```python
from build123d import *

# Parameters (mm, degrees)
PAD_DEPTH       = 23
POCKET_DEPTH    = 20
SKETCH002_R     = 3
PAD001_DEPTH    = 5
SKETCH003_R     = 1.75
POCKET001_DEPTH = 7
SKETCH004_R     = 7
POCKET002_DEPTH = 37


with BuildPart() as part:
    # Sketch (on Face1 of ShapeBinder) → Pad (new body)
    with BuildSketch(Plane.XY.offset(1.6)):
        with BuildLine():
            Line((65.104061, -85.85), (78.671175, -85.849875))
            ThreePointArc((78.671175, -85.849875), (81.499513, -84.678339), (82.67105, -81.850001))
            ThreePointArc((85.065002, -79.425001), (83.370362, -80.146209), (82.67105, -81.850001))
            Line((85.065002, -79.425001), (184.315, -79.425))
            Line((184.315, -79.425), (184.315, -33.325))
            Line((184.315, -33.325), (85.065, -33.325))
            Line((85.065, -33.325), (66.055583, -33.325))
            Line((66.055583, -33.325), (58.318648, -33.167991))
            ThreePointArc((58.318648, -33.167991), (41.347688, -32.282578), (32.59625, -46.85))
            Line((32.59625, -46.85), (32.59625, -81.85))
            ThreePointArc((32.59625, -81.85), (47.081166, -98.22649), (65.104061, -85.85))
        make_face()
    extrude(amount=PAD_DEPTH)

    # Sketch001 (on Face11 of Pad) → Pocket (cut)
    with BuildSketch(Plane.XY.offset(24.6)):
        with BuildLine():
            Line((85.065004, -76.42489), (181.315, -76.425))
            Line((181.315, -76.425), (181.315, -36.325))
            Line((181.315, -36.325), (66.055583, -36.325))
            ThreePointArc((66.055583, -36.325), (66.025147, -36.324846), (65.994715, -36.324382))
            Line((65.994715, -36.324382), (58.25778, -36.167373))
            ThreePointArc((58.25778, -36.167373), (57.41292, -36.028001), (56.641848, -35.655629))
            ThreePointArc((56.641848, -35.655629), (42.756517, -34.9312), (35.59625, -46.85))
            Line((35.59625, -46.85), (35.59625, -81.85))
            ThreePointArc((35.59625, -81.85), (47.447597, -95.248953), (62.193575, -85.122625))
            ThreePointArc((62.193575, -85.122625), (63.25771, -83.485372), (65.104092, -82.849876))
            Line((65.104092, -82.849876), (78.671175, -82.849878))
            ThreePointArc((78.671175, -82.849878), (79.378193, -82.557021), (79.67105, -81.850003))
            ThreePointArc((85.065004, -76.42489), (81.249022, -78.024869), (79.67105, -81.850003))
        make_face()
    extrude(amount=-POCKET_DEPTH, mode=Mode.SUBTRACT)

    # Sketch002 (on Face26 of Pocket) → Pad001 (join)
    with BuildSketch(Plane.XY.offset(4.6)):
        with Locations((64.665, -78.375)):
            Circle(SKETCH002_R)
        with Locations((49.065, -64.325)):
            Circle(SKETCH002_R)
        with Locations((60.665, -41.375)):
            Circle(SKETCH002_R)
        with Locations((104.065, -56.325)):
            Circle(SKETCH002_R)
        with Locations((123.165, -56.375)):
            Circle(SKETCH002_R)
        with Locations((142.215, -56.375)):
            Circle(SKETCH002_R)
        with Locations((161.265, -56.375)):
            Circle(SKETCH002_R)
    extrude(amount=PAD001_DEPTH)

    # Sketch003 (on Face37 of Pad001) → Pocket001 (cut)
    with BuildSketch(Plane.XY.offset(9.6)):
        with Locations((49.065, -64.325)):
            Circle(SKETCH003_R)
        with Locations((64.665, -78.375)):
            Circle(SKETCH003_R)
        with Locations((60.665, -41.375)):
            Circle(SKETCH003_R)
        with Locations((142.215, -56.375)):
            Circle(SKETCH003_R)
        with Locations((161.265, -56.375)):
            Circle(SKETCH003_R)
        with Locations((104.065, -56.325)):
            Circle(SKETCH003_R)
        with Locations((123.165, -56.375)):
            Circle(SKETCH003_R)
    extrude(amount=-POCKET001_DEPTH, mode=Mode.SUBTRACT)

    # Sketch004 → Pocket002 (cut)
    with BuildSketch(Plane.XZ):
        with Locations((72.507256, 16.6)):
            Circle(SKETCH004_R)
    extrude(amount=POCKET002_DEPTH, mode=Mode.SUBTRACT)


solid = part.part
```
Source: CAD feature listing. Evaluate the final solid. Frame: model axes, mm. A direction names the side the tool comes from. Coordinates: 2 decimals unless noted, no trailing zeros. Loops run counter-clockwise (first coordinate to the right, second up) from the corner with the lowest first, then second, coordinate; pieces in that order, holes last. Notation, with made-up numbers: M -3.75,-33 L 38.25,-33 A26 cw 38.25,3 Z; hole C 77,13 d6. An arc over 180 degrees is marked long. Put each result on its own line as item: value. Start each with the question number.
1) Cut plane B-B on z = 16.6. Return the cut outline in (x, y) (3 decimals), then the cut area to 3 significant figures.
2) Reachability of faces 1 (the face through (65.514, -34.797, 16.908)), 2 (the face through (46.75, -98.182, 12.939)), 3 (the face through (144, -58, 9.6)), 4 (the face through (126, -33.325, 13)) from +Z, -Z, +X, -X, +Y, -Y: full face, straight path, thin tool, end or side. Return the list, or none.
3) Cut plane A-A on y = -51.5. Return the cut outline in (x, z) (3 decimals), then the cut area to 3 significant figures.
4) Cut plane C-C on x = 128. Return the cut outline in (y, z) (3 decimals), then the cut area to 3 significant figures.
5) Pull-direction query (Y, two-part tool) for faces 5 (the face through (97, -77, 24.6)), 6 (the face through (81.47, -84.71, 12.94)), 7 (the face through (41.569, -32.167, 12.939)), 8 (the face through (65, -78, 2.6)); classes: pulls with the +Y half, pulls with the -Y half, needs draft (parallel to the pull), parting line crosses it, or undercut.
6) Contact query for flat-ended pins moving along their axis: pin 1 Ø10 at (x, z) = (113.5, 10) entering from -Y (3 decimals); pin 2 Ø5 at (x, y) = (160, -56) entering from +Z; pin 3 Ø1 at (x, y) = (143, -56.5) entering from +Z. Output: stop coordinate, or through.
7) Ray query, L1, parallel to Y at x = 134.5, z = 22.5 (3 decimals); L2, parallel to X at y = -69, z = 21.5 (3 decimals); L3, parallel to X at y = -35, z = 14 (3 decimals). Return the intervals inside material, ascending. Write a range as from..to.
The answers:
1. outline: M 32.596,-81.85 A16.5 ccw 65.104,-85.85 L 78.671,-85.85 A4 ccw 82.671,-81.85 A2.425 cw 85.065,-79.425 L 184.315,-79.425 L 184.315,-33.325 L 79.507,-33.325 L 79.507,-36.325 L 181.315,-36.325 L 181.315,-76.425 L 85.065,-76.425 A5.425 ccw 79.671,-81.85 A1 cw 78.671,-82.85 L 65.104,-82.85 A3 ccw 62.194,-85.123 A13.5 cw 35.596,-81.85 L 35.596,-46.85 A13.5 cw 56.642,-35.656 A3 ccw 58.258,-36.167 L 65.507,-36.314 L 65.507,-33.314 L 58.319,-33.168 A16.5 ccw 32.596,-46.85 Z
1. area: 1,170 mm²
2. face 1: +Y
2. face 2: +Z, -Z, -Y
2. face 3: +Z
2. face 4: +Z, -Z, +X, +Y
3. outline: M 32.596,1.6 L 184.315,1.6 L 184.315,24.6 L 181.315,24.6 L 181.315,4.6 L 35.596,4.6 L 35.596,24.6 L 32.596,24.6 Z
3. area: 575 mm²
4. outline: M -79.425,1.6 L -33.325,1.6 L -33.325,24.6 L -36.325,24.6 L -36.325,4.6 L -76.425,4.6 L -76.425,24.6 L -79.425,24.6 Z
4. area: 258 mm²
5. face 5: needs draft
5. face 6: pulls with the -Y half
5. face 7: pulls with the +Y half
5. face 8: undercut
6. pin 1: stops at y = -79.425
6. pin 2: stops at z = 9.6
6. pin 3: stops at z = 2.6
7. L1: y = -79.425..-76.425, -36.325..-33.325
7. L2: x = 32.596..35.596, 181.315..184.315
7. L3: x = 37.615..42.629, 55.564..66.008, 79.006..184.315
